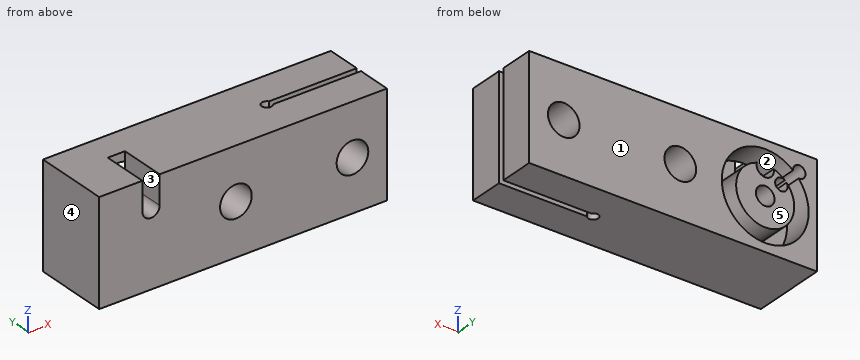
Autodesk Inventor part; units mm, degrees
ref_plane "YZ Plane" through (0, 0, 0) normal (1, 0, 0) x (0, 1, 0)
ref_plane "XZ Plane" through (0, 0, 0) normal (0, 1, 0) x (-1, 0, 0)
ref_plane "XY Plane" through (0, 0, 0) normal (0, 0, 1) x (1, 0, 0)
sketch "Sketch1" plane through (0, 0, 0) normal (0, 0, 1) x (1, 0, 0)
  line L0 (-25, -6.5) -> (25, -6.5)
  line L1 (25, -6.5) -> (25, 6.5)
  line L2 (25, 6.5) -> (-25, 6.5)
  line L3 (-25, 6.5) -> (-25, -6.5)
  line L4 (-25, -6.5) -> (25, 6.5) construction
  line L5 (25, -6.5) -> (-25, 6.5) construction
  line L6 (25, 0) -> (9, 0)
  circle A0 centre (9, 0) radius 0.89
  line L7 (25, 0) -> (25, 0.5)
  line L8 (25, 0.5) -> (9.7363, 0.5)
  line L9 (25, 0) -> (25, -0.5)
  line L10 (25, -0.5) -> (9.7363, -0.5)
  point P0 (0, 0)
  dimension "d0" = 50
  dimension "d1" = 13
  dimension "d2" = 16
  dimension "d3" = 1.78
  dimension "d4" = 0.5
  dimension "d5" = 0.5
extrude "Extrusion1" add sketch "Sketch1" against normal blind 18 contours L3 L2 L1 L8 A0 L10 L0
sketch "Sketch2" plane through (-25, -6.5, 0) normal (0, -1, 0) x (1, 0, 0)
  line L0 (50, 0) -> (50, -18)
  line L1 (50, -9) -> (44, -9)
  line L2 (44, -9) -> (23.75, -9)
  circle A0 centre (44, -9) radius 4.375
  circle A1 centre (23.75, -9) radius 4.375
  line L3 (0, 0) -> (7.5, 0)
  line L4 (50, 0) -> (0, 0)
  line L5 (7.5, 0) -> (9, 0)
  line L6 (9, 0) -> (9, -5)
  circle A2 centre (9, -5) radius 1.5
  line L7 (7.5, 0) -> (7.5, -5)
  line L8 (9, 0) -> (10.5, 0)
  line L9 (10.5, 0) -> (10.5, -5)
  point P0 (25, 0)
  dimension "d8" = 6
  dimension "d9" = 20.25
  dimension "d10" = 8.75
  dimension "d11" = 8.75
  dimension "d12" = 7.5
  dimension "d13" = 1.5
  dimension "d14" = 5
  dimension "d15" = 3
hole "Hole1" at (19, -6.5, -9) at (-1.25, -6.5, -9) direction (0, 1, 0) diameter 5.5 end through all
extrude "Extrusion2" cut sketch "Sketch2" against normal blind 8 contours L9 A2 L6 L4 | L6 A2 L7 L4 | A2
sketch "Sketch3" plane through (-25, 6.5, 0) normal (0, 1, 0) x (1, 0, 0)
  line L0 (0, 0) -> (0, 18)
  line L1 (0, 0) -> (18, 18)
  line L2 (0, 18) -> (50, 18)
  line L3 (0, 0) -> (25.4558, 0) construction
  circle A0 centre (9, 9) radius 7.55
  circle A1 centre (9, 9) radius 5.05
  circle A2 centre (9, 9) radius 2
  line L4 (9, 7) -> (9, 4.5)
  circle A3 centre (9, 4.5) radius 1.5
  line L5 (5.4291, 5.4291) -> (6.1857, 6.1857)
  circle A4 centre (6.1857, 6.1857) radius 1.085
  line L6 (0, 0) -> (3.085, 3.085)
  circle A5 centre (3.085, 3.085) radius 1.085
  point P0 (25, 0)
  point P1 (4.1636, 3.2024)
  point P2 (3.2024, 4.1636)
  point P3 (7.5376, 4.1664)
  point P4 (5.5752, 5.2888)
  point P5 (5.2888, 5.5752)
  point P6 (10.4624, 4.1664)
  dimension "d27" = 10.1
  dimension "d28" = 4
  dimension "d25" = 45
  dimension "d26" = 15.1
  dimension "d29" = 2.5
  dimension "d30" = 3
  dimension "d31" = 1.07
  dimension "d32" = 2.17
  dimension "d33" = 4.3628
  dimension "d34" = 2.17
extrude "Extrusion3" cut sketch "Sketch3" against normal blind 5 contours A0 L1 A1 A4 A5 | A0 A5 L1 A4 A1 A3 | A3 A1 | A1 A3
hole "Hole2" at (-16, 6.5, -9) direction (0, -1, 0) diameter 3.242 depth 8.5 tip angle 118
hole "Hole3" at (-18.8143, 6.5, -6.1857) at (-21.915, 6.5, -3.085) direction (0, -1, 0) diameter 2.17 depth 8.5
properties part number "levelmeter-top"
Design review of the part built by this model. Coordinates are the model's own, in mm. Face numbers are marked on the shaded views. A direction names the side the tool comes from. Round coordinates to 2 decimals unless told otherwise and drop trailing zeros. Write each loop counter-clockwise with the first axis right and the second up, starting at its lowest first coordinate (ties: lowest second). Pieces come first, ordered by that corner, then holes.
Item 1: We need section D-D on x = -2.5. Write out the cut boundary in (y, z), and give its area (3 significant figures).
Item 2: For the marked faces 1 and 2, list the 3-axis set-ups (+Z, -Z, +X, -X, +Y, -Y) from which the entire face can be reached by the end or side of a thin tool; tool diameter is ignored.
Item 3: We need section B-B on x = 9. Write out the cut boundary in (y, z).
Item 4: We need section C-C on y = -3.5. Write out the cut boundary in (x, z), and give its area (3 significant figures).
Item 5: We need section A-A on y = 2.5. Write out the cut boundary in (x, z) (3 decimals).
Item 6: Clearance check with a flat-ended pin moving along its axis: pin 1 Ø0.7 at (x, z) = (-19, -6.5) entering from +Y. State where the tip first meets the part, or that it passes through.
Item 7: The part is to be moulded in two halves that separate along X. For the marked faces 3, 4 and 5, say which applies: +X half, -X half, draft (parallel to the pull), parting line (faces both ways), or undercut.
Item 8: For probe 1 along Z at (x, y) = (-16, 3.5); probe 2 along Y at (x, z) = (9, -5); probe 3 along X at (y, z) = (2.25, -10), list the stretches that pass through material, from the lowest coordinate up.
Returned:
1. outline: (-6.5, -18) - (6.5, -18) - (6.5, -11.45) - (-6.5, -11.45) - close; (-6.5, -6.55) - (6.5, -6.55) - (6.5, 0) - (-6.5, 0) - close
1. area: 170 mm2
2. face 1: +Z, -Z, +X, -X, +Y
2. face 2: +Y
3. outline: (-6.5, -18) - (-0.89, -18) - (-0.89, 0) - (-6.5, 0) - close; (0.89, -18) - (6.5, -18) - (6.5, 0) - (0.89, 0) - close
4. outline: (-25, -18) - (25, -18) - (25, 0) - (-14.5, 0) - (-14.5, -5) arc R1.5 cw to (-17.5, -5) - (-17.5, 0) - (-25, 0) - close; hole circle Ø5.5 at (-1.25, -9); hole circle Ø5.5 at (19, -9)
4. area: 834 mm2
5. outline: (-25, -18) - (25, -18) - (25, 0) - (-25, 0) - close; (-19.711, -5.575) arc R5.05 ccw (long way) to (-14.538, -4.166) arc R1.5 cw (long way) to (-17.462, -4.166) arc R5.05 ccw to (-19.425, -5.289) arc R1.085 cw (long way) to start; hole (-21.798, -4.164) arc R7.55 ccw (long way) to (-20.836, -3.202) arc R1.085 ccw (long way) to start; hole circle Ø3.242 at (-16, -9); hole circle Ø5.5 at (-1.25, -9); hole circle Ø5.5 at (19, -9)
6. pin 1: stops at y = -2
7. face 3: undercut
7. face 4: -X half
7. face 5: draft
8. probe 1: z = -18 to -16.55, -14.05 to -10.62, -7.38 to -6, -1.45 to 0
8. probe 2: y = -6.5 to -0.89, 0.89 to 6.5
8. probe 3: x = -25 to -23.48, -20.95 to -17.28, -14.72 to -11.05, -8.52 to -3.81, 1.31 to 16.44, 21.56 to 25
